For this review, take the finished solid that the model builds, in its own axes (mm). A direction names the side the tool comes from. Coordinates: 2 decimals unless noted, no trailing zeros. Order: outer loops, then holes, each group sorted by start corner. A loop starts at its lowest first (then second) coordinate and runs counter-clockwise, first axis right, second up. Notation, with made-up numbers: (52, 83) -> (66, 83) arc R30 cw to (66, 108) -> close; hole circle Ø2 at (-26.75, 60.25). An arc over 180 degrees is marked (long way). Answer as a JSON object with one key per item and string values. Group by question number.
1) Add section C-C, the plane y = -2. Count the separate pieces of the cut face and the enclosed holes in it, then the cut area to 3 significant figures.
2) Wall thickness on L1, parallel to X at y = -5, z = -17.5; L2, parallel to Z at x = -32, y = -0.25; L3, parallel to Z at x = -26, y = -3.5: over which ranges is each line inside the solid? List them lowest first.
3) Add section A-A, the plane x = -48.5. Write out the cut boundary in (y, z).
4) Add section B-B, the plane z = 0. Write out the cut boundary in (x, y).
5) For pin 1 (3 mm diameter, centred on x = -26, y = -4.5, fed in from +Z); pin 2 (1 mm diameter, centred on y = -1.5, z = -19.5, fed in from -X); pin 3 (1.5 mm diameter, centred on x = -43, y = -2, fed in from +Z), all flat-tipped, find the tip position at first contact; note any pin that passes through.
6) Machinability: for faces 1 (the cylindrical face through (-35, -3, 1.7)), 2 (the flat face through (-34, -6, -8)), which of the approach directions +Z, -Z, +X, -X, +Y, -Y give a long, thin tool a straight path to every point of the face, cutting with its end or side? Answer none if there is none.
7) Draft analysis for pull direction X (two halves, no side actions). For faces 3 (the cylindrical face through (-28.518, -2.958, 9.505)), 4 (the cylindrical face through (-47.622, -3.042, -24.224)), 5 (the cylindrical face through (-32.284, -3.042, 12.634)), state which applies: +X half, -X half, draft (parallel to the pull), parting line (faces both ways), or undercut.
8) Add section D-D, the plane z = -11. Write out the cut boundary in (x, y).
from build123d import *

# Parameters (mm, degrees)
RESSALTO_EXTRUS_O1_DEPTH = 6
CORTE_EXTRUS_O1_DEPTH    = 7.0000001
CORTE_EXTRUS_O2_DEPTH    = 7.0000001
CORTE_EXTRUS_O3_DEPTH    = 7.0000001
CORTE_EXTRUS_O4_DEPTH    = 7.0000001
ESBO_O6_R                = 1.6
CORTE_EXTRUS_O5_DEPTH    = 7.0000001
ESBO_O7_R                = 1.6
CORTE_EXTRUS_O6_DEPTH    = 7.0000001


with BuildPart() as part:
    # Esboço1 → Ressalto-extrusão1 (new body)
    with BuildSketch(Plane.XZ.offset(6)):
        with BuildLine():
            Line((-35.053391166, -1.665767354), (-56.005959689, -18.507024557))
            ThreePointArc((-56.005959689, -18.507024557), (-56.976417823, -19.646228266), (-57.460270003, -21.062371319))
            ThreePointArc((-57.460270003, -21.062371319), (-56.122071197, -23.520718894), (-53.5, -24.5))
            Line((-53.5, -24.5), (-49.26036734, -24.5))
            ThreePointArc((-49.26036734, -24.5), (-47.599906261, -24.216234622), (-46.127917729, -23.397147602))
            Line((-46.127917729, -23.397147602), (-18.051593362, -0.829957358))
            ThreePointArc((-18.051593362, -0.829957358), (-16.213367114, 2.526467109), (-17.286895371, 6.199639856))
            ThreePointArc((-17.286895371, 6.199639856), (-17.752824847, 6.738395184), (-18.256300836, 7.242239912))
            ThreePointArc((-18.256300836, 7.242239912), (-18.528297677, 7.80831066), (-18.343735303, 8.408606506))
            add(Edge.make_bspline(
                [(-18.343735303, 8.408606506), (-16.98173735, 9.54416389), (-17.156613946, 12.29450716)],
                knots=[0.078549619, 0.078549619, 0.078549619, 0.770539159, 0.770539159, 0.770539159], degree=2, weights=[1, 0.940738559, 1]))
            ThreePointArc((-17.156613946, 12.29450716), (-32.291666667, 12.629537139), (-39.569048555, -0.645317995))
            add(Edge.make_bspline(
                [(-39.569048555, -0.645317995), (-37.274619711, -2.171937204), (-35.610199193, -1.560191069)],
                knots=[2.371053495, 2.371053495, 2.371053495, 3.063043035, 3.063043035, 3.063043035], degree=2, weights=[1, 0.940738559, 1]))
            ThreePointArc((-35.610199193, -1.560191069), (-35.322864942, -1.565881251), (-35.053391166, -1.665767354))
        make_face()
    extrude(amount=-RESSALTO_EXTRUS_O1_DEPTH)

    # Esboço2 → Corte-extrusão1 (cut, through all)
    with BuildSketch(Plane(origin=(0, 0, 0), x_dir=(-1, 0, 0), z_dir=(0, 1, 0))):
        with BuildLine():
            ThreePointArc((24.354682005, 14.569048555), (21.225555592, 14.0864183), (18.274337499, 12.939825155))
            add(Edge.make_bspline(
                [(21.046065504, 9.968797575), (20.743642938, 11.716101094), (18.274337499, 12.939825155)],
                knots=[3.220142273, 3.220142273, 3.220142273, 3.912131812, 3.912131812, 3.912131812], degree=2, weights=[1, 0.940738559, 1]))
            ThreePointArc((21.046065504, 9.968797575), (21.47365577, 9.508813947), (22.099885838, 9.461334748))
            ThreePointArc((22.099885838, 9.461334748), (22.438769866, 9.558640989), (22.780905164, 9.643813326))
            ThreePointArc((22.780905164, 9.643813326), (23.299496712, 9.998046554), (23.439808931, 10.610199193))
            add(Edge.make_bspline(
                [(24.354682005, 14.569048555), (22.828062796, 12.274619711), (23.439808931, 10.610199193)],
                knots=[2.371053495, 2.371053495, 2.371053495, 3.063043035, 3.063043035, 3.063043035], degree=2, weights=[1, 0.940738559, 1]))
        make_face()
    extrude(amount=-CORTE_EXTRUS_O1_DEPTH, mode=Mode.SUBTRACT)

    # Esboço3 → Corte-extrusão2 (cut, through all)
    with BuildSketch(Plane(origin=(0, 0, 0), x_dir=(-1, 0, 0), z_dir=(0, 1, 0))):
        with BuildLine():
            ThreePointArc((31.725662501, 12.939825155), (28.774444408, 14.0864183), (25.645317995, 14.569048555))
            add(Edge.make_bspline(
                [(26.560191069, 10.610199193), (27.171937204, 12.274619711), (25.645317995, 14.569048555)],
                knots=[3.220142273, 3.220142273, 3.220142273, 3.912131812, 3.912131812, 3.912131812], degree=2, weights=[1, 0.940738559, 1]))
            ThreePointArc((26.560191069, 10.610199193), (26.700503288, 9.998046554), (27.219094836, 9.643813326))
            ThreePointArc((27.219094836, 9.643813326), (27.561230134, 9.558640989), (27.900114162, 9.461334748))
            ThreePointArc((27.900114162, 9.461334748), (28.52634423, 9.508813947), (28.953934496, 9.968797575))
            add(Edge.make_bspline(
                [(31.725662501, 12.939825155), (29.256357062, 11.716101094), (28.953934496, 9.968797575)],
                knots=[2.371053495, 2.371053495, 2.371053495, 3.063043035, 3.063043035, 3.063043035], degree=2, weights=[1, 0.940738559, 1]))
        make_face()
    extrude(amount=-CORTE_EXTRUS_O2_DEPTH, mode=Mode.SUBTRACT)

    # Esboço4 → Corte-extrusão3 (cut, through all)
    with BuildSketch(Plane(origin=(0, 0, 0), x_dir=(-1, 0, 0), z_dir=(0, 1, 0))):
        with BuildLine():
            ThreePointArc((37.29450716, 7.843386054), (35.311973892, 10.311973892), (32.843386054, 12.29450716))
            add(Edge.make_bspline(
                [(31.656264697, 8.408606506), (33.01826265, 9.54416389), (32.843386054, 12.29450716)],
                knots=[3.220142273, 3.220142273, 3.220142273, 3.912131812, 3.912131812, 3.912131812], degree=2, weights=[1, 0.940738559, 1]))
            ThreePointArc((31.656264697, 8.408606506), (31.471702323, 7.80831066), (31.743699164, 7.242239912))
            ThreePointArc((31.743699164, 7.242239912), (31.997410855, 6.997410855), (32.242239912, 6.743699164))
            ThreePointArc((32.242239912, 6.743699164), (32.80831066, 6.471702323), (33.408606506, 6.656264697))
            add(Edge.make_bspline(
                [(37.29450716, 7.843386054), (34.54416389, 8.01826265), (33.408606506, 6.656264697)],
                knots=[5.512646149, 5.512646149, 5.512646149, 6.204635688, 6.204635688, 6.204635688], degree=2, weights=[1, 0.940738559, 1]))
        make_face()
    extrude(amount=-CORTE_EXTRUS_O3_DEPTH, mode=Mode.SUBTRACT)

    # Esboço5 → Corte-extrusão4 (cut, through all)
    with BuildSketch(Plane(origin=(0, 0, 0), x_dir=(-1, 0, 0), z_dir=(0, 1, 0))):
        with BuildLine():
            ThreePointArc((39.569048555, 0.645317995), (39.0864183, 3.774444408), (37.939825155, 6.725662501))
            add(Edge.make_bspline(
                [(34.968797575, 3.953934496), (36.716101094, 4.256357062), (37.939825155, 6.725662501)],
                knots=[3.220142273, 3.220142273, 3.220142273, 3.912131812, 3.912131812, 3.912131812], degree=2, weights=[1, 0.940738559, 1]))
            ThreePointArc((34.968797575, 3.953934496), (34.508813947, 3.52634423), (34.461334748, 2.900114162))
            ThreePointArc((34.461334748, 2.900114162), (34.558640989, 2.561230134), (34.643813326, 2.219094836))
            ThreePointArc((34.643813326, 2.219094836), (34.998046554, 1.700503288), (35.610199193, 1.560191069))
            add(Edge.make_bspline(
                [(39.569048555, 0.645317995), (37.274619711, 2.171937204), (35.610199193, 1.560191069)],
                knots=[2.371053495, 2.371053495, 2.371053495, 3.063043035, 3.063043035, 3.063043035], degree=2, weights=[1, 0.940738559, 1]))
        make_face()
    extrude(amount=-CORTE_EXTRUS_O4_DEPTH, mode=Mode.SUBTRACT)

    # Esboço6 → Corte-extrusão5 (cut, through all)
    with BuildSketch(Plane.XZ.offset(6)):
        with Locations((-25, 0)):
            Circle(ESBO_O6_R)
    extrude(amount=-CORTE_EXTRUS_O5_DEPTH, mode=Mode.SUBTRACT)

    # Esboço7 → Corte-extrusão6 (cut, through all)
    with BuildSketch(Plane(origin=(0, 0, 0), x_dir=(-1, 0, 0), z_dir=(0, 1, 0))):
        with Locations((47.598401843, -18.16414524)):
            Circle(ESBO_O7_R)
    extrude(amount=-CORTE_EXTRUS_O6_DEPTH, mode=Mode.SUBTRACT)


solid = part.part
Output values:
{
 "1": {"separate pieces": "1", "enclosed holes": "2", "area": "576 mm²"},
 "2": {"L1": "x = -54.75 to -49.05, -46.14 to -38.79", "L2": "z = -12.04 to 6.99, 8.76 to 12.79", "L3": "z = -7.22 to -1.25, 1.25 to 13.99"},
 "3": {"outline": "(-6, -24.44) -> (0, -24.44) -> (0, -19.49) -> (-6, -19.49) -> close; (-6, -16.84) -> (0, -16.84) -> (0, -12.47) -> (-6, -12.47) -> close"},
 "4": {"outline": "(-39.58, -6) -> (-26.6, -6) -> (-26.6, 0) -> (-39.58, 0) -> close; (-23.4, -6) -> (-17.24, -6) -> (-17.24, 0) -> (-23.4, 0) -> close"},
 "5": {"pin 1": "stops at z = 14.58", "pin 2": "stops at x = -57.16", "pin 3": "stops at z = -7.45"},
 "6": {"face 1": "+Y, -Y", "face 2": "+Z, -Z, +X, -X, -Y"},
 "7": {"face 3": "undercut", "face 4": "+X half", "face 5": "-X half"},
 "8": {"outline": "(-46.67, -6) -> (-30.7, -6) -> (-30.7, 0) -> (-46.67, 0) -> close"}
}
